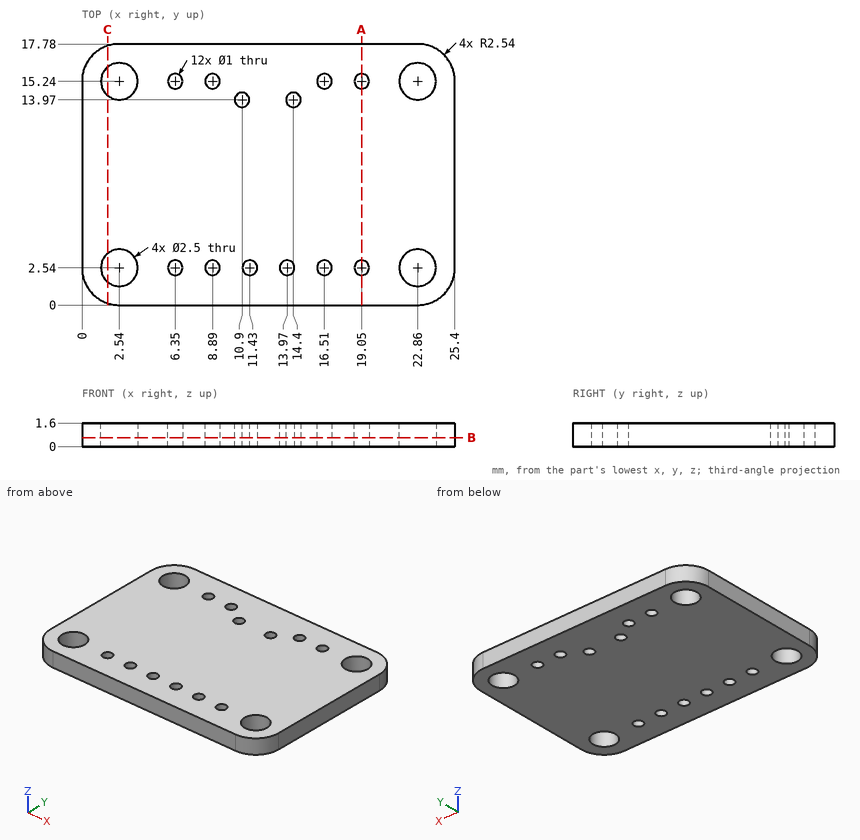
Could you check a few things on this drawing? It's one solid part, dimensions in mm from its lowest x, y, z. Round coordinates to 2 decimals unless told otherwise and drop trailing zeros. Loops run counter-clockwise (first coordinate to the right, second up) from the corner with the lowest first, then second, coordinate; pieces in that order, holes last. Notation, with made-up numbers: (41.5, 17) -> (97.5, 17) arc R15 cw to (97.5, 37) -> close; hole circle Ø5 at (9, 11). An arc over 180 degrees is marked (long way). One line per item, written item: value. Start each with the question number.
1. For pin 1 (2 mm diameter, centred on x = 2.54, y = 2.54, fed in from +Z), with a flat end and sliding along its axis, tell me the tip position at first contact or that it passes through.
2. If we section it at B-B, the plane z = 0.6: Give the number of separate pieces and of enclosed holes in the cut face, then the cut area to 3 significant figures.
3. If we section it at C-C, the plane x = 1.75: Write out the boundary of the cut face in (y, z).
4. If I drill on probe 1 along Y at (x, z) = (16.51, 0.95); probe 2 along X at (y, z) = (14.5, 1.2); probe 3 along Y at (x, z) = (6.75, 0.15), over which ranges is the centre line in solid material (lowest first)?
5. If we section it at A-A, the plane x = 19.05: Write out the boundary of the cut face in (y, z), then the cut area to 3 significant figures.
Calculated:
1. pin 1: passes through
2. separate pieces: 1
2. enclosed holes: 16
2. area: 417 mm²
3. outline: (0.13, 0) -> (1.57, 0) -> (1.57, 1.6) -> (0.13, 1.6) -> close; (3.51, 0) -> (14.27, 0) -> (14.27, 1.6) -> (3.51, 1.6) -> close; (16.21, 0) -> (17.65, 0) -> (17.65, 1.6) -> (16.21, 1.6) -> close
4. probe 1: y = 0 to 2.04, 3.04 to 14.74, 15.74 to 17.78
4. probe 2: x = 0 to 1.53, 3.55 to 21.85, 23.87 to 25.4
4. probe 3: y = 0 to 2.24, 2.84 to 14.94, 15.54 to 17.78
5. outline: (0, 0) -> (2.04, 0) -> (2.04, 1.6) -> (0, 1.6) -> close; (3.04, 0) -> (14.74, 0) -> (14.74, 1.6) -> (3.04, 1.6) -> close; (15.74, 0) -> (17.78, 0) -> (17.78, 1.6) -> (15.74, 1.6) -> close
5. area: 25.2 mm²
